from build123d import *

# Parameters (mm, degrees)
SKETCH1_R           = 1
SKETCH1_R_2         = 2
BOSS_EXTRUDE1_DEPTH = 3


with BuildPart() as part:
    # Sketch1 → Boss-Extrude1 (new body)
    with BuildSketch(Plane(origin=(0, 0, 0), x_dir=(1, 0, 0), z_dir=(0, 1, 0))):
        with BuildLine():
            Line((64.190973866, -16.340444348), (48.133067619, -16.340444348))
            Line((48.133067619, -16.340444348), (48.133067619, -13.340444349))
            Line((48.133067619, -13.340444349), (64.190973866, -13.340444349))
            ThreePointArc((64.190973866, -13.340444349), (60.864318365, -6.794408764), (54.189826358, -3.733628612))
            ThreePointArc((54.189826358, -3.733628612), (53.662670154, -3.708804342), (53.135527124, -3.683701873))
            ThreePointArc((53.135527124, -3.683701873), (24.702146142, -1.915932839), (-3.669341235, 0.661054823))
            ThreePointArc((-3.669341235, 0.661054823), (-5.346030709, 0.838891836), (-7.022417949, 1.019555652))
            ThreePointArc((-7.022417949, 1.019555652), (-22.882417949, -14.840444348), (-7.022417949, -30.700444348))
            ThreePointArc((-7.022417949, -30.700444348), (-5.346030709, -30.519780533), (-3.669341235, -30.341943519))
            ThreePointArc((-3.669341235, -30.341943519), (24.702146142, -27.764955858), (53.135527124, -25.997186824))
            ThreePointArc((53.135527124, -25.997186824), (53.662670154, -25.972084355), (54.189826358, -25.947260084))
            ThreePointArc((54.189826358, -25.947260084), (60.864318365, -22.886479933), (64.190973866, -16.340444348))
        make_face()
        with Locations((-19.472417949, -14.840444348)):
            Circle(SKETCH1_R, mode=Mode.SUBTRACT)
        with Locations((-13.247417949, -14.840444348)):
            Circle(SKETCH1_R, mode=Mode.SUBTRACT)
        with Locations((-7.022417949, -14.840444348)):
            Circle(SKETCH1_R_2, mode=Mode.SUBTRACT)
        with Locations((-0.797417949, -14.840444348)):
            Circle(SKETCH1_R, mode=Mode.SUBTRACT)
        with Locations((5.427582051, -14.840444348)):
            Circle(SKETCH1_R, mode=Mode.SUBTRACT)
    extrude(amount=BOSS_EXTRUDE1_DEPTH)


solid = part.part
Work out the finished part from the listing and answer in its coordinate system (mm). A direction names the side the tool comes from. Give positions to 0.01 mm unless a question says otherwise; leave off trailing zeros. Loops run counter-clockwise (first coordinate to the right, second up) from the corner with the lowest first, then second, coordinate; pieces in that order, holes last. Notation, with made-up numbers: (73, 3) -> (90, 3) arc R10 ccw to (90, 16) -> close; hole circle Ø5 at (65.25, 7.5). An arc over 180 degrees is marked (long way). Use a Markdown table: item, result. Add a question column.
1. For faces 1 (the flat face through (56, 1, 16.34)), 2 (the cylindrical face through (-7.46, 1.48, 16.79)), determine the directions among +Z, -Z, +X, -X, +Y, -Y from which every point of the face is accessible in a straight line to the end or side of a thin tool.
2. Section D-D on x = 49 is taken. Determine the outline of the cut face in (y, z).
3. Section A-A on x = 58 is taken. Determine the outline of the cut face in (y, z).
4. Find the intervals of material crossed by probe 1 along X at (y, z) = (2.65, 15); probe 2 along Z at (x, y) = (60, 2.75); probe 3 along Z at (x, y) = (59, 0.6), in increasing order.
5. Determine the mould class of faces 3 (the cylindrical face through (5.211, 1.479, 15.817)), 4 (the cylindrical face through (-5.37, 1.479, 30.522)), 5 (the cylindrical face through (25.1, 1.479, 1.946)) for opening direction Z: released by +Z, released by -Z, zero draft, split by the parting line, or undercut.
6. Flat-ended cylindrical pins translate along their axes: pin 1 Ø3 at (x, z) = (-7.02, 14.84) entering from -Y; pin 2 Ø0.9 at (x, y) = (52.5, 1.5) entering from -Z; pin 3 Ø0.9 at (y, z) = (2, 15) entering from +X. Find the tip coordinate at first contact, or state that the pin passes through.
7. Section B-B on y = 0.9 is taken. Determine the outline of the cut face in (x, z), and give its area (3 significant figures).
8. Section C-C on z = 23.5 is taken. Determine the outline of the cut face in (x, y).
Results below:
| question | item | result |
|---|---|---|
| 1 | face 1 | +X, +Y, -Y |
| 1 | face 2 | +Y, -Y |
| 2 | outline | (0, 3.48) -> (3, 3.48) -> (3, 13.34) -> (0, 13.34) -> close; (0, 16.34) -> (3, 16.34) -> (3, 26.2) -> (0, 26.2) -> close |
| 3 | outline | (0, 4.8) -> (3, 4.8) -> (3, 13.34) -> (0, 13.34) -> close; (0, 16.34) -> (3, 16.34) -> (3, 24.88) -> (0, 24.88) -> close |
| 4 | probe 1 | x = -22.88 to -20.46, -18.49 to -14.23, -12.26 to -9.02, -5.03 to -1.78, 0.19 to 4.44, 6.41 to 48.13 |
| 4 | probe 2 | z = 6.05 to 13.34, 16.34 to 23.64 |
| 4 | probe 3 | z = 5.35 to 13.34, 16.34 to 24.33 |
| 5 | face 3 | undercut |
| 5 | face 4 | released by +Z |
| 5 | face 5 | released by -Z |
| 6 | pin 1 | passes through |
| 6 | pin 2 | stops at z = 3.63 |
| 6 | pin 3 | stops at x = 48.13 |
| 7 | outline | (-7.02, -1.02) arc R1000 cw to (-3.67, -0.66) arc R1000 cw to (53.14, 3.68) arc R1000 cw to (54.19, 3.73) arc R11.16 ccw to (64.19, 13.34) -> (48.13, 13.34) -> (48.13, 16.34) -> (64.19, 16.34) arc R11.16 ccw to (54.19, 25.95) arc R1000 cw to (53.14, 26) arc R1000 cw to (-3.67, 30.34) arc R1000 cw to (-7.02, 30.7) arc R15.86 ccw to start; hole circle Ø2 at (-19.47, 14.84); hole circle Ø2 at (-13.25, 14.84); hole circle Ø4 at (-7.02, 14.84); hole circle Ø2 at (-0.8, 14.84); hole circle Ø2 at (5.43, 14.84) |
| 7 | area | 2,110 mm^2 |
| 8 | outline | (-20.31, 0) -> (60.17, 0) -> (60.17, 3) -> (-20.31, 3) -> close |
